The listing builds one solid part. Answer for the finished solid, in the listing's coordinates (mm). A direction names the side the tool comes from. Round coordinates to 2 decimals unless told otherwise and drop trailing zeros. Write each loop counter-clockwise with the first axis right and the second up, starting at its lowest first coordinate (ties: lowest second). Pieces come first, ordered by that corner, then holes.
(1) Find the intervals of material crossed by probe 1 along X at (y, z) = (35, -6); probe 2 along Y at (x, z) = (34.5, 5.5); probe 3 along Y at (x, z) = (15.5, -1.5), in increasing order.
(2) A cutting plane is placed at B-B, the plane z = 1.5. Give the vertices of the cut face in (x, y).
(3) For faces 4 (the face through (4.5, 5, 6)), 5 (the face through (-22, 4, 5.185)), 6 (the face through (-22, 1, -0.985)), 7 (the face through (-19.998, 24.906, -5.988)), 8 (the face through (-37.5, 37, -7)), determine the directions among +Z, -Z, +X, -X, +Y, -Y from which every point of the face is accessible in a straight line to the end or side of a thin tool.
(4) Each of these flat-tipped pins is pushed along its axis until it touches: pin 1 Ø1 at (x, z) = (-25, 6) entering from +Y; pin 2 Ø1 at (x, z) = (2, 6) entering from +Y. Where does it stop, or does it pass through?
(5) A cutting plane is placed at C-C, the plane x = -25.5. Give the vertices of the cut face in (y, z) (3 decimals).
(6) A cutting plane is placed at D-D, the plane y = 11.5. Give the vertices of the cut face in (x, z) (3 decimals), and give its area (3 significant figures).
(7) A cutting plane is placed at A-A, the plane x = 0. Give the vertices of the cut face in (y, z) (3 decimals).
(8) The mould has two halves that part along Y. Classify faces 1 (the face through (-38, 1, 1)), 2 (the face through (-20, 3.81, -5.06)), 3 (the face through (-1, 0, -1)): +Y half, -Y half, draft (parallel to the pull), parting line (faces both ways), or undercut.
from build123d import *

# Parameters (mm, degrees)
CROQUIS1_W              = 79
CROQUIS1_H              = 14.37
SALIENTE_EXTRUIR1_DEPTH = 2
SALIENTE_EXTRUIR2_DEPTH = 79
CROQUIS4_W              = 35
CROQUIS4_H              = 2
SALIENTE_EXTRUIR3_DEPTH = 5
CORTAR_EXTRUIR1_REACH   = 66.124
CROQUIS5_W              = 9
CROQUIS5_H              = 9.995566824
CORTAR_EXTRUIR2_REACH   = 68.213
CROQUIS6_W              = 35.5
CROQUIS6_H              = 21.095495938
CROQUIS6_H_2            = 21.095495939
CORTAR_EXTRUIR3_REACH   = 66.124
CROQUIS7_W              = 32
CROQUIS7_H              = 4.169878309
SALIENTE_EXTRUIR4_REACH = 70.495
CROQUIS8_W              = 2
CROQUIS8_H              = 2
SALIENTE_EXTRUIR5_REACH = 70.495
CROQUIS11_W             = 2
CROQUIS11_H             = 2


with BuildPart() as part:
    # Croquis1 → Saliente-Extruir1 (new body)
    with BuildSketch(Plane(origin=(0, 0, 0), x_dir=(1, 0, 0), z_dir=(0, 1, 0))):
        Rectangle(CROQUIS1_W, CROQUIS1_H)
    extrude(amount=SALIENTE_EXTRUIR1_DEPTH)

    # Croquis2 → Saliente-Extruir2 (add)
    with BuildSketch(Plane(origin=(39.5, 0, 0), x_dir=(0, 0, -1), z_dir=(1, 0, 0))):
        Polygon((2.810566824, 2), (7.185, 52), (7.185, 2), align=None)
    extrude(amount=-SALIENTE_EXTRUIR2_DEPTH)

    # Croquis4 → Saliente-Extruir3 (add)
    with BuildSketch(Plane(origin=(0, 2, 0), x_dir=(1, 0, 0), z_dir=(0, 1, 0))):
        with Locations((-22, -6.185)):
            Rectangle(CROQUIS4_W, CROQUIS4_H)
    saliente_extruir3 = extrude(amount=SALIENTE_EXTRUIR3_DEPTH)

    # Simetría1: Saliente-Extruir3 across plane
    add(saliente_extruir3.mirror(Plane(origin=(0, 0, 0), x_dir=(0, 0, 1), z_dir=(1, 0, 0))))

    # Croquis5 → Cortar-Extruir1 (cut, up to next)
    with BuildSketch(Plane(origin=(0, 2, 0), x_dir=(1, 0, 0), z_dir=(0, 1, 0)), mode=Mode.PRIVATE) as cortar_extruir1_sk1:
        with Locations((0, -2.187216588)):
            Rectangle(CROQUIS5_W, CROQUIS5_H)
    cortar_extruir1_tool1 = extrude(cortar_extruir1_sk1.sketch, amount=-CORTAR_EXTRUIR1_REACH, mode=Mode.PRIVATE) & part.part
    add(cortar_extruir1_tool1.solids().sort_by_distance((0, 2, 2.187217))[0], mode=Mode.SUBTRACT)

    # Cortar-Extruir2: up to this plane
    cortar_extruir2_end = Plane(origin=(39.5, 2, -7.185), z_dir=(0, 0, 1))
    # Croquis6 → Cortar-Extruir2 (cut, up to the surface)
    with BuildSketch(Plane(origin=(0, -0.228832657, -2.615569233), x_dir=(1, 0, 0), z_dir=(0, 0.0871557427476544, 0.996194698091746)), mode=Mode.PRIVATE) as cortar_extruir2_sk1:
        with Locations((-19.75, 39.880590343)):
            Rectangle(CROQUIS6_W, CROQUIS6_H)
    cortar_extruir2_tool1 = split(extrude(cortar_extruir2_sk1.sketch, amount=-CORTAR_EXTRUIR2_REACH, mode=Mode.PRIVATE), bisect_by=cortar_extruir2_end, keep=Keep.BOTH, mode=Mode.PRIVATE)
    add(cortar_extruir2_tool1.solids().sort_by_distance((-19.75, 39.5, -6.091392))[0], mode=Mode.SUBTRACT)
    # Croquis6 → Cortar-Extruir2 (cut, up to the surface)
    with BuildSketch(Plane(origin=(0, -0.228832657, -2.615569233), x_dir=(1, 0, 0), z_dir=(0, 0.0871557427476544, 0.996194698091746)), mode=Mode.PRIVATE) as cortar_extruir2_sk2:
        with Locations((19.75, 39.880590343)):
            Rectangle(CROQUIS6_W, CROQUIS6_H)
    cortar_extruir2_tool2 = split(extrude(cortar_extruir2_sk2.sketch, amount=-CORTAR_EXTRUIR2_REACH, mode=Mode.PRIVATE), bisect_by=cortar_extruir2_end, keep=Keep.BOTH, mode=Mode.PRIVATE)
    add(cortar_extruir2_tool2.solids().sort_by_distance((19.75, 39.5, -6.091392))[0], mode=Mode.SUBTRACT)
    # Croquis6 → Cortar-Extruir2 (cut, up to the surface)
    with BuildSketch(Plane(origin=(0, -0.228832657, -2.615569233), x_dir=(1, 0, 0), z_dir=(0, 0.0871557427476544, 0.996194698091746)), mode=Mode.PRIVATE) as cortar_extruir2_sk3:
        with Locations((19.75, 14.785094405)):
            Rectangle(CROQUIS6_W, CROQUIS6_H_2)
    cortar_extruir2_tool3 = split(extrude(cortar_extruir2_sk3.sketch, amount=-CORTAR_EXTRUIR2_REACH, mode=Mode.PRIVATE), bisect_by=cortar_extruir2_end, keep=Keep.BOTH, mode=Mode.PRIVATE)
    add(cortar_extruir2_tool3.solids().sort_by_distance((19.75, 14.5, -3.904175))[0], mode=Mode.SUBTRACT)
    # Croquis6 → Cortar-Extruir2 (cut, up to the surface)
    with BuildSketch(Plane(origin=(0, -0.228832657, -2.615569233), x_dir=(1, 0, 0), z_dir=(0, 0.0871557427476544, 0.996194698091746)), mode=Mode.PRIVATE) as cortar_extruir2_sk4:
        with Locations((-19.75, 14.785094405)):
            Rectangle(CROQUIS6_W, CROQUIS6_H_2)
    cortar_extruir2_tool4 = split(extrude(cortar_extruir2_sk4.sketch, amount=-CORTAR_EXTRUIR2_REACH, mode=Mode.PRIVATE), bisect_by=cortar_extruir2_end, keep=Keep.BOTH, mode=Mode.PRIVATE)
    add(cortar_extruir2_tool4.solids().sort_by_distance((-19.75, 14.5, -3.904175))[0], mode=Mode.SUBTRACT)

    # Croquis7 → Cortar-Extruir3 (cut, up to next)
    with BuildSketch(Plane(origin=(0, 2, 0), x_dir=(1, 0, 0), z_dir=(0, 1, 0)), mode=Mode.PRIVATE) as cortar_extruir3_sk1:
        with Locations((22, -1.100060846)):
            Rectangle(CROQUIS7_W, CROQUIS7_H)
    cortar_extruir3_tool1 = extrude(cortar_extruir3_sk1.sketch, amount=-CORTAR_EXTRUIR3_REACH, mode=Mode.PRIVATE) & part.part
    cortar_extruir3 = cortar_extruir3_tool1.solids().sort_by_distance((22, 2, 1.100061))[0]
    add(cortar_extruir3, mode=Mode.SUBTRACT)

    # Simetría4: Cortar-Extruir3 across plane
    add(cortar_extruir3.mirror(Plane(origin=(0, 0, 0), x_dir=(0, 0, 1), z_dir=(1, 0, 0))), mode=Mode.SUBTRACT)

    # Croquis8 → Saliente-Extruir4 (add, up to next)
    with BuildSketch(Plane(origin=(-4.5, 0, 0), x_dir=(0, 0, -1), z_dir=(1, 0, 0)), mode=Mode.PRIVATE) as saliente_extruir4_sk1:
        with Locations((-6.185, 1)):
            Rectangle(CROQUIS8_W, CROQUIS8_H)
    saliente_extruir4_tool1 = extrude(saliente_extruir4_sk1.sketch, amount=SALIENTE_EXTRUIR4_REACH, mode=Mode.PRIVATE) - part.part
    add(saliente_extruir4_tool1.solids().sort_by_distance((-4.5, 1, 6.185))[0])

    # Croquis11 → Saliente-Extruir5 (add, up to next)
    with BuildSketch(Plane(origin=(-4.5, 0, 0), x_dir=(0, 0, -1), z_dir=(1, 0, 0)), mode=Mode.PRIVATE) as saliente_extruir5_sk1:
        with Locations((1.810566824, 1)):
            Rectangle(CROQUIS11_W, CROQUIS11_H)
    saliente_extruir5_tool1 = extrude(saliente_extruir5_sk1.sketch, amount=SALIENTE_EXTRUIR5_REACH, mode=Mode.PRIVATE) - part.part
    add(saliente_extruir5_tool1.solids().sort_by_distance((-4.5, 1, -1.810567))[0])


solid = part.part
Solutions:
1. probe 1: x = -39.5 to -37.5, -2 to 2, 37.5 to 39.5
1. probe 2: y = 0 to 7
1. probe 3: y = 0 to 2
2. outline: (-39.5, 0) - (-38, 0) - (-38, 2) - (-39.5, 2) - close; (-6, 0) - (-4.5, 0) - (-4.5, 2) - (-6, 2) - close; (4.5, 0) - (6, 0) - (6, 2) - (4.5, 2) - close; (38, 0) - (39.5, 0) - (39.5, 2) - (38, 2) - close
3. face 4: +Z, +Y
3. face 5: +X, -X, +Y
3. face 6: +Y, -Y
3. face 7: +Z
3. face 8: +Z, -Z
4. pin 1: stops at y = 7
4. pin 2: stops at y = 2
5. outline: (0, -7.185) - (3.625, -7.185) - (3.992, -2.985) - (2, -2.811) - (2, -0.985) - (0, -0.985) - close; (0, 3.185) - (2, 3.185) - (2, 5.185) - (7, 5.185) - (7, 7.185) - (0, 7.185) - close; (24.801, -7.185) - (28.816, -7.185) - (28.992, -5.172) - (25.008, -4.823) - close; (49.992, -7.185) - (52, -7.185) - (50.008, -7.011) - close
6. outline: (-39.5, -7.185) - (-37.5, -7.185) - (-37.5, -3.642) - (-39.5, -3.642) - close; (-2, -7.185) - (2, -7.185) - (2, -3.642) - (-2, -3.642) - close; (37.5, -7.185) - (39.5, -7.185) - (39.5, -3.642) - (37.5, -3.642) - close
6. area: 28.3 mm2
7. outline: (0, -7.185) - (52, -7.185) - (2, -2.811) - (2, -0.811) - (0, -0.811) - close; (0, 5.185) - (2, 5.185) - (2, 7.185) - (0, 7.185) - close
8. face 1: draft
8. face 2: undercut
8. face 3: -Y half
